Input: part model. Units: mm. Frame: model coordinates. A direction names the side the tool comes from. Give positions to 0.01 mm unless a question says otherwise; leave off trailing zeros. Loops run counter-clockwise (first coordinate to the right, second up) from the corner with the lowest first, then second, coordinate; pieces in that order, holes last. Notation, with made-up numbers: (-12.5, 12.25) -> (6.5, 12.25) arc R27 cw to (6.5, 34.25) -> close; hole circle Ø1 at (40, 50.25). An arc over 180 degrees is marked (long way). Answer as a JSON object with one key per item and string values.
```python
from build123d import *

# Parameters (mm, degrees)
CYLINDER033_R          = 1.6
CYLINDER033_DEPTH      = 10
CYLINDER033_ROLL_ANGLE = -90
CYLINDER032_R          = 1.6
CYLINDER032_DEPTH      = 10
CYLINDER032_ROLL_ANGLE = -90
BOX029_W               = 3
BOX029_H               = 10
BOX029_DEPTH           = 22
BOX031_W               = 4
BOX031_H               = 7
BOX031_DEPTH           = 22
BOX030_W               = 26
BOX030_H               = 3
BOX030_DEPTH           = 21
CHAMFER006_SIZE        = 12
BOX028_W               = 61
BOX028_H               = 3
BOX028_DEPTH           = 10
CHAMFER007_SIZE        = 3
FILLET026_R            = 1


with BuildPart() as cylinder033:
    # Cylinder033 → Cylinder033 (new body)
    with BuildSketch(Plane.XY):
        Circle(CYLINDER033_R)
    extrude(amount=CYLINDER033_DEPTH)


with BuildPart() as cylinder033_1:
    # Cylinder033 roll: moved
    add(cylinder033.part.rotate(Axis((0, 0, 0), (1, 0, 0)), CYLINDER033_ROLL_ANGLE))


with BuildPart() as cylinder033_2:
    # Cylinder033 placement: moved
    add(cylinder033_1.part.moved(Location((-15.5, 30, 38.5))))


with BuildPart() as fusion029:
    # Cylinder032 → Cylinder032 (new body)
    with BuildSketch(Plane.XY):
        Circle(CYLINDER032_R)
    extrude(amount=CYLINDER032_DEPTH)


with BuildPart() as fusion029_1:
    # Cylinder032 roll: moved
    add(fusion029.part.rotate(Axis((0, 0, 0), (1, 0, 0)), CYLINDER032_ROLL_ANGLE))


with BuildPart() as fusion029_2:
    # Cylinder032 placement: moved
    add(fusion029_1.part.moved(Location((-44.5, 30, 38.5))))

    # Fusion029: union Cylinder033
    add(cylinder033_2.part)


with BuildPart() as cube029:
    # Box029 → Box029 (new body)
    with BuildSketch(Plane(origin=(-73, 35, 20), x_dir=(1, 0, 0), z_dir=(0, 0, 1))):
        with Locations((1.5, 5)):
            Rectangle(BOX029_W, BOX029_H)
    extrude(amount=BOX029_DEPTH)


with BuildPart() as cube031:
    # Box031 → Box031 (new body)
    with BuildSketch(Plane(origin=(-61, 30, 20), x_dir=(1, 0, 0), z_dir=(0, 0, 1))):
        with Locations((2, 3.5)):
            Rectangle(BOX031_W, BOX031_H)
    extrude(amount=BOX031_DEPTH)


with BuildPart() as chamfer006:
    # Box030 → Box030 (new body)
    with BuildSketch(Plane(origin=(-71, 35, 20), x_dir=(1, 0, 0), z_dir=(0, 0, 1))):
        with Locations((13, 1.5)):
            Rectangle(BOX030_W, BOX030_H)
    extrude(amount=BOX030_DEPTH)

    # Chamfer006
    chamfer006_edges = [chamfer006.edges().sort_by_distance(p)[0] for p in [
        (-45, 36.5, 20),
    ]]
    chamfer(chamfer006_edges, length=CHAMFER006_SIZE)


with BuildPart() as fillet026:
    # Box028 → Box028 (new body)
    with BuildSketch(Plane(origin=(-71, 35, 32), x_dir=(1, 0, 0), z_dir=(0, 0, 1))):
        with Locations((30.5, 1.5)):
            Rectangle(BOX028_W, BOX028_H)
    extrude(amount=BOX028_DEPTH)

    # Fusion026: union Chamfer006
    add(chamfer006.part)

    # Fusion027: union Cube031
    add(cube031.part)

    # Fusion028: union Cube029
    add(cube029.part)

    # Chamfer007
    chamfer007_edges = [fillet026.edges().sort_by_distance(p)[0] for p in [
        (-61, 32.5, 42),
    ]]
    chamfer(chamfer007_edges, length=CHAMFER007_SIZE)

    # Cut037: cut Fusion029
    add(fusion029_2.part, mode=Mode.SUBTRACT)

    # Fillet026
    fillet026_edges = [fillet026.edges().sort_by_distance(p)[0] for p in [
        (-10, 36.5, 32),
        (-70, 38, 31),
    ]]
    fillet(fillet026_edges, radius=FILLET026_R)


solid = fillet026.part
```
Q1. Section B-B, the plane z = 29. Return the cut outline in (x, y), then the cut area to 3 significant figures.
Evaluation:
{"outline": "(-73, 35) -> (-61, 35) -> (-61, 30) -> (-57, 30) -> (-57, 35) -> (-48, 35) -> (-48, 38) -> (-69, 38) arc R1 cw to (-70, 39) -> (-70, 45) -> (-73, 45) -> close", "area": "116 mm2"}
Q2. Ray query, line 1 along Z through (x, y) = (-44.5, 36.1); line 2 along X through (y, z) = (44.25, 34); line 3 along Y through (x, z) = (-49, 30.25). Return the intervals inside material, ascending.
Evaluation:
{"line 1": "z = 32 to 36.9, 40.1 to 42", "line 2": "x = -73 to -70", "line 3": "y = 35 to 38"}
Q3. Section C-C, the plane y = 31.75. Return the cut outline in (x, z), then the cut area to 3 significant figures.
Evaluation:
{"outline": "(-61, 20) -> (-57, 20) -> (-57, 42) -> (-58, 42) -> (-61, 39) -> close", "area": "83.5 mm2"}
Q4. Section A-A, the plane x = -15.5. Return the cut outline in (y, z), then the cut area to 3 significant figures.
Evaluation:
{"outline": "(35, 32) -> (38, 32) -> (38, 36.9) -> (35, 36.9) -> close; (35, 40.1) -> (38, 40.1) -> (38, 42) -> (35, 42) -> close", "area": "20.4 mm2"}
Q5. Section D-D, the plane x = -43.5. Return the cut outline in (y, z), then the cut area to 3 significant figures.
Evaluation:
{"outline": "(35, 32) -> (38, 32) -> (38, 37.25) -> (35, 37.25) -> close; (35, 39.75) -> (38, 39.75) -> (38, 42) -> (35, 42) -> close", "area": "22.5 mm2"}
Q6. Access query for faces 1 (the flat face through (-57, 32, 31)), 2 (the flat face through (-70, 42, 31)), 3 (the flat face through (-28, 37, 32)). Directions: +Z, -Z, +X, -X, +Y, -Y. A direction counts if a zero-diameter tool reaches every point of the face in a straight line with its end or side. Return the directions, or none.
Evaluation:
{"face 1": "+Z, -Z, +X, -Y", "face 2": "+Z, -Z, +X, +Y", "face 3": "-Z, +X, +Y, -Y"}
Q7. Pin query (flat end, axial travel): pin 1 (4.5 mm diameter, centred on x = -68, z = 29, fed in from -Y); pin 2 (10 mm diameter, centred on x = -44, z = 35.5, fed in from +Y); pin 3 (1 mm diameter, centred on x = -45.5, y = 36, fed in from -Z). Return the tip coordinate at first contact, or that it passes through.
Evaluation:
{"pin 1": "stops at y = 35", "pin 2": "stops at y = 38", "pin 3": "stops at z = 31"}
Q8. Draft query along X for faces 4 (the cylindrical face through (-16.77, 36.48, 39.47)), 5 (the flat face through (-34, 35, 36)), 6 (the flat face through (-51, 36, 26)). Return one class per face: +X half, -X half, draft (parallel to the pull), parting line (faces both ways), or undercut.
Evaluation:
{"face 4": "undercut", "face 5": "draft", "face 6": "+X half"}
